```python
from build123d import *

# Parameters (mm, degrees)
IZIM1_R                     = 12.5
IZIM1_R_2                   = 1.5
Y_KSEKLIK_EKSTR_ZYON1_DEPTH = 3
IZIM2_R                     = 7
IZIM2_R_2                   = 5
EKSTR_ZYON_NCE1_DEPTH       = 10
IZIM3_R                     = 1.5
KES_EKSTR_ZYON1_DEPTH       = 22.943108257
IZIM2_2_R                   = 5
KES_EKSTR_ZYON2_DEPTH       = 21.310096061


with BuildPart() as part:
    # izim1 → Y_kseklik-Ekstr_zyon1 (new body)
    with BuildSketch(Plane(origin=(0, 0, 0), x_dir=(1, 0, 0), z_dir=(0, 1, 0))):
        with Locations(Location((0, 0, 0), (0, 0, 270))):
            Circle(IZIM1_R)
        with Locations(Location((10, 0, 0), (0, 0, 270))):
            Circle(IZIM1_R_2, mode=Mode.SUBTRACT)
        with Locations(Location((0, -10, 0), (0, 0, 270))):
            Circle(IZIM1_R_2, mode=Mode.SUBTRACT)
        with Locations(Location((-10, 0, 0), (0, 0, 270))):
            Circle(IZIM1_R_2, mode=Mode.SUBTRACT)
        with Locations(Location((0, 10, 0), (0, 0, 270))):
            Circle(IZIM1_R_2, mode=Mode.SUBTRACT)
    extrude(amount=Y_KSEKLIK_EKSTR_ZYON1_DEPTH)

    # izim2 → Ekstr_zyon-_nce1 (add)
    with BuildSketch(Plane(origin=(0, 3, 0), x_dir=(1, 0, 0), z_dir=(0, 1, 0))):
        Circle(IZIM2_R)
        Circle(IZIM2_R_2, mode=Mode.SUBTRACT)
    extrude(amount=EKSTR_ZYON_NCE1_DEPTH)

    # izim3 → Kes-Ekstr_zyon1 (cut, through all)
    with BuildSketch(Plane(origin=(0, 0, 0), x_dir=(0, 0, -1), z_dir=(1, 0, 0))):
        with Locations((0, 8)):
            Circle(IZIM3_R)
    extrude(amount=-KES_EKSTR_ZYON1_DEPTH, mode=Mode.SUBTRACT)

    # izim2_2 → Kes-Ekstr_zyon2 (cut, through all)
    with BuildSketch(Plane(origin=(0, 3, 0), x_dir=(1, 0, 0), z_dir=(0, 1, 0))):
        with Locations(Location((0, 0, 0), (0, 0, 270))):
            Circle(IZIM2_2_R)
    extrude(amount=-KES_EKSTR_ZYON2_DEPTH, mode=Mode.SUBTRACT)


solid = part.part
```
CAD build for the part. Positions are in the model's coordinates, mm. A direction names the side the tool comes from. Round coordinates to 2 decimals unless told otherwise and drop trailing zeros. Order: outer loops, then holes, each group sorted by start corner. A loop starts at its lowest first (then second) coordinate and runs counter-clockwise, first axis right, second up.
Q1. Which spindle directions (+Z, -Z, +X, -X, +Y, -Y) get a long thin tool onto all of the face, cutting with end or side? Do faces 4 (the cylindrical face through (-5.9, 7.1, 1.2)), 5 (the cylindrical face through (0.07, 1.48, -11.5)), 6 (the flat face through (-5.4, 3, 5.4)). Say none if no direction does.
Q2. Two-plate mould, pull along X, no slides. Class faces 1 (the cylindrical face through (0.07, 1.48, 8.5)), 2 (the flat face through (-5.4, 0, -0.2)), 3 (the cylindrical face through (3.755, 1.479, 11.923)): pulls with the +X half, pulls with the -X half, needs draft (parallel to the pull), parting line crosses it, or undercut.
Q3. Slice it at B-B (x = 0). Write the cut outline in (y, z).
Q4. Slice it at A-A (z = -10). Write the cut outline in (x, y).
Q5. Drop flat-ended pins along their axis: pin 1 (2.5 mm diameter, centred on x = 0, z = 10, fed in from +Y); pin 2 (4 mm diameter, centred on x = 0, z = -10, fed in from +Y); pin 3 (1 mm diameter, centred on x = 6, y = 9.5, fed in from -Z); pin 4 (1.5 mm diameter, centred on y = 9, z = -6, fed in from +X). Give the stop position or say it passes through.
Q6. Slice it at D-D (x = -10). Write the cut outline in (y, z).
Q7. Slice it at C-C (z = 0). Write the cut outline in (x, y), and give its area (3 significant figures).
Q8. Wall check: L1, parallel to X at y = 1.3, z = 0; L2, parallel to X at y = 3.25, z = 0; L3, parallel to Y at x = -5.4, z = 0. Give the ranges that are in metal, low to high.
Results below:
1. face 4: -X
1. face 5: +Y, -Y
1. face 6: +Y
2. face 1: undercut
2. face 2: needs draft
2. face 3: parting line crosses it
3. outline: (0, -12.5) - (3, -12.5) - (3, -11.5) - (0, -11.5) - close; (0, -8.5) - (3, -8.5) - (3, -7) - (13, -7) - (13, -5) - (0, -5) - close; (0, 5) - (13, 5) - (13, 7) - (3, 7) - (3, 8.5) - (0, 8.5) - close; (0, 11.5) - (3, 11.5) - (3, 12.5) - (0, 12.5) - close
4. outline: (-7.5, 0) - (-1.5, 0) - (-1.5, 3) - (-7.5, 3) - close; (1.5, 0) - (7.5, 0) - (7.5, 3) - (1.5, 3) - close
5. pin 1: passes through
5. pin 2: stops at y = 3
5. pin 3: stops at z = -4.33
5. pin 4: stops at x = 4.63
6. outline: (0, -7.5) - (3, -7.5) - (3, -1.5) - (0, -1.5) - close; (0, 1.5) - (3, 1.5) - (3, 7.5) - (0, 7.5) - close
7. outline: (-12.5, 0) - (-11.5, 0) - (-11.5, 3) - (-12.5, 3) - close; (-8.5, 0) - (-5, 0) - (-5, 6.5) - (-7, 6.5) - (-7, 3) - (-8.5, 3) - close; (-7, 9.5) - (-5, 9.5) - (-5, 13) - (-7, 13) - close; (5, 0) - (8.5, 0) - (8.5, 3) - (7, 3) - (7, 13) - (5, 13) - close; (11.5, 0) - (12.5, 0) - (12.5, 3) - (11.5, 3) - close
7. area: 61.0 mm2
8. L1: x = -12.5 to -11.5, -8.5 to -5, 5 to 8.5, 11.5 to 12.5
8. L2: x = -7 to -5, 5 to 7
8. L3: y = 0 to 6.5, 9.5 to 13
